Geometry: see drawing. Coordinates: mm, zero at the bounding-box minimum. Coordinates: 2 decimals unless noted, no trailing zeros. Order: outer loops, then holes, each group sorted by start corner. A loop starts at its lowest first (then second) coordinate and runs counter-clockwise, first axis right, second up. Notation, with made-up numbers: M 81.25,78 L 130.25,78 A23 cw 130.25,115 Z; hole C -5,-38 d9. An arc over 180 degrees is marked long. Answer in a Markdown table with one row per item.
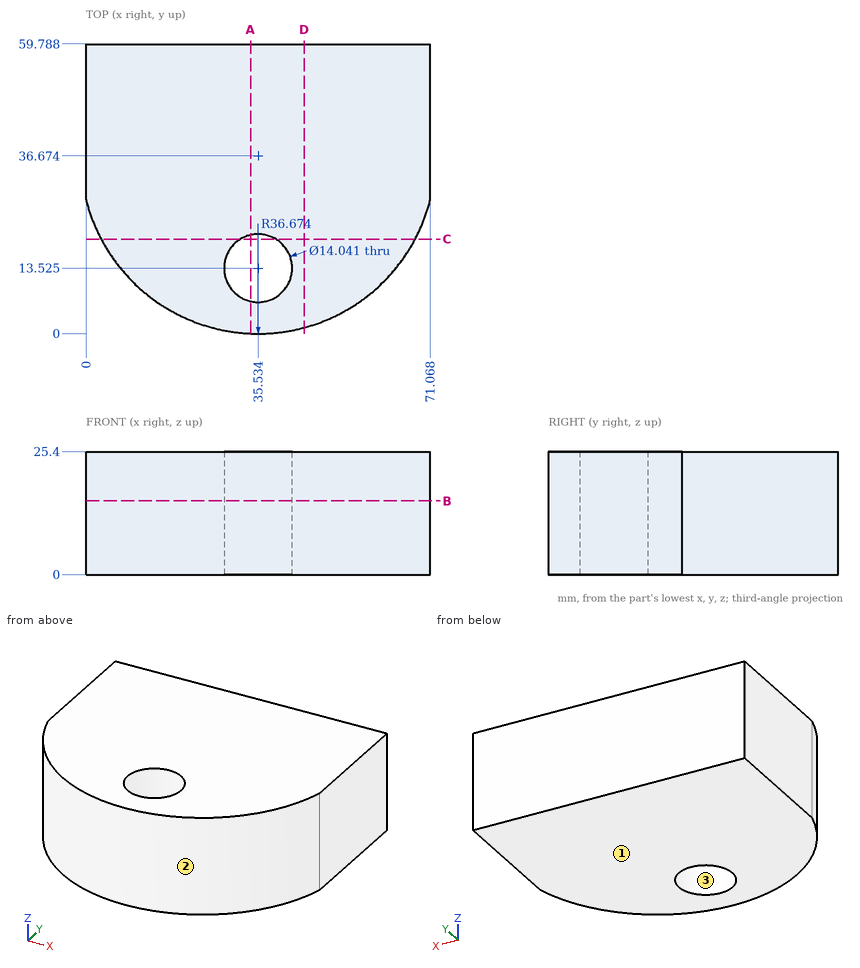
1) Material intervals for probe 1 along Y at (x, z) = (33, 14.75); probe 2 along X at (y, z) = (19, 21) (1 decimal); probe 3 along Y at (x, z) = (30, 14) (1 decimal), sorted ascending.
Resolved:
| item | result |
|---|---|
| probe 1 | y = 0.09 to 6.98, 20.07 to 59.79 |
| probe 2 | x = 3.4 to 31.1, 39.9 to 67.7 |
| probe 3 | y = 0.4 to 9.2, 17.8 to 59.8 |
2) Cut plane C-C, the plane y = 19.5. Output: boundary loops of the cut face in (x, z).
Resolved:
| item | result |
|---|---|
| outline | M 3.13,0 L 31.85,0 L 31.85,25.4 L 3.13,25.4 Z; M 39.22,0 L 67.94,0 L 67.94,25.4 L 39.22,25.4 Z |
3) Contact query for flat-ended pins moving along their axis: pin 1 (1 mm diameter, centred on x = 8, z = 8.5, fed in from -Y); pin 2 (5 mm diameter, centred on x = 62, z = 6, fed in from -Y) (1 decimal); pin 3 (1.5 mm diameter, centred on x = 9.5, z = 18, fed in from -Y). Output: stop coordinate, or through.
Resolved:
| item | result |
|---|---|
| pin 1 | stops at y = 11.89 |
| pin 2 | stops at y = 8.9 |
| pin 3 | stops at y = 10.11 |
4) Cut plane D-D, the plane x = 45. Output: boundary loops of the cut face in (y, z), and give its area (3 significant figures).
Resolved:
| item | result |
|---|---|
| outline | M 1.24,0 L 59.79,0 L 59.79,25.4 L 1.24,25.4 Z |
| area | 1,490 mm2 |
5) Cut plane A-A, the plane x = 34. Output: boundary loops of the cut face in (y, z) (1 decimal), and give its area (3 significant figures).
Resolved:
| item | result |
|---|---|
| outline | M 0,0 L 6.7,0 L 6.7,25.4 L 0,25.4 Z; M 20.4,0 L 59.8,0 L 59.8,25.4 L 20.4,25.4 Z |
| area | 1,170 mm2 |
6) Cut plane B-B, the plane z = 15.25. Output: boundary loops of the cut face in (x, y) (1 decimal), and give its area (3 significant figures).
Resolved:
| item | result |
|---|---|
| outline | M 0,27.6 A36.7 ccw 71.1,27.6 L 71.1,59.8 L 0,59.8 Z; hole C 35.5,13.5 d14 |
| area | 3,590 mm2 |
7) Mould query, pull axis Y, two halves, no side actions, for the marked faces 1, 2 and 3. Classes: +Y half, -Y half, draft (parallel to the pull), parting line (faces both ways), or undercut.
Resolved:
| item | result |
|---|---|
| face 1 | draft |
| face 2 | -Y half |
| face 3 | undercut |
